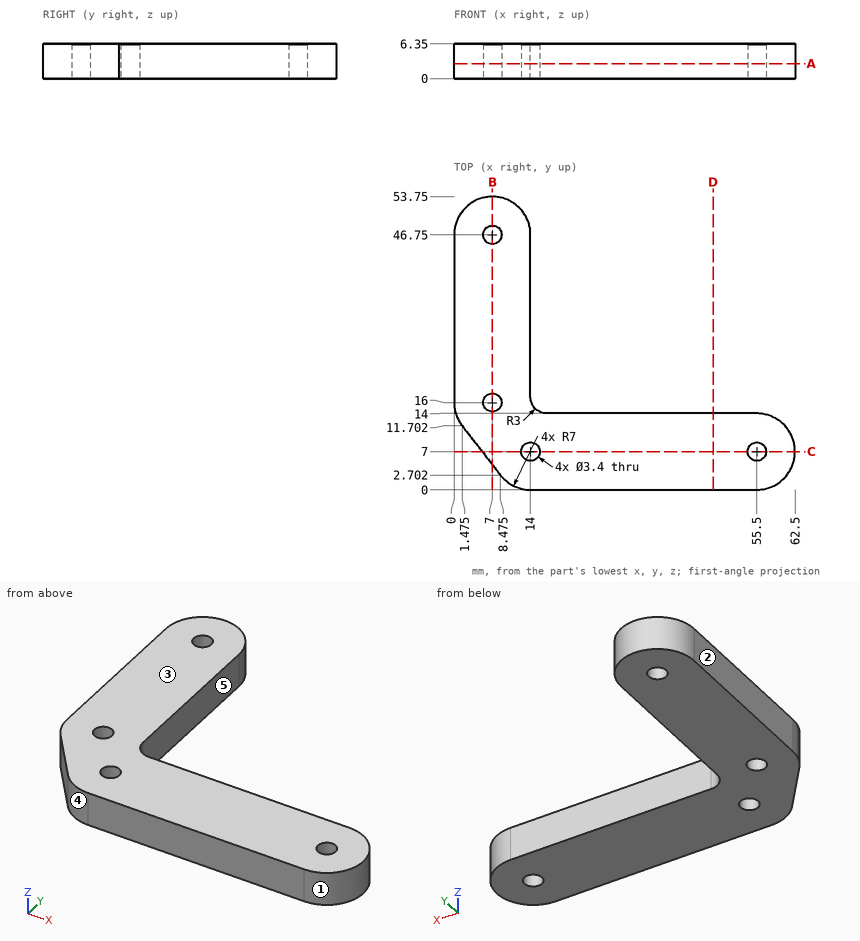
Answer from the drawing. Dimensions are ordinates in mm from the lowest x, y and z of the part. A direction names the side the tool comes from. Coordinates: 2 decimals unless noted, no trailing zeros. Write each loop counter-clockwise with the first axis right and the second up, starting at its lowest first coordinate (ties: lowest second). Pieces come first, ordered by that corner, then holes. Notation, with made-up numbers: M 38,49 L 61,49 A12 ccw 61,56 Z; hole C 38,88.5 d9. An arc over 180 degrees is marked long. Put each result on its own line as item: value. Start each with the question number.
1. Consider line 1 (Y direction, x = 32.5, z = 1.5); line 2 (Y direction, x = 14.5, z = 5) (1 decimal). Determine where each line is inside the solid, lowest interval first. Write a range as from..to.
2. A cutting plane is placed at B-B on x = 7. Write down the section's boundary in (y, z), then the cut area to 3 significant figures.
3. Which of the six approach directions +Z, -Z, +X, -X, +Y, -Y give full straight-line access (tool end or side, diameter ignored) to the marked faces 4 and 5?
4. A flat-ended cylindrical pin translates along its axis: P1, Ø3, axis at x = 26, z = 1, coming from the +Y side. Find the tip coordinate at first contact, or state that the pin passes through.
5. A cutting plane is placed at A-A on z = 2.75. Count the separate pieces of the cut face and the enclosed holes in it, then the cut area to 3 significant figures.
6. A cutting plane is placed at C-C on y = 7. Write down the section's boundary in (x, z).
7. For a pull along X with two mould halves and no side action, classify the marked faces 1, 2 and 3 as pulls with the +X half, pulls with the -X half, needs draft (parallel to the pull), parting line crosses it, or undercut.
8. A cutting plane is placed at D-D on x = 47.5. Write down the section's boundary in (y, z), then the cut area to 3 significant figures.
Resolved:
1. line 1: y = 0..14
1. line 2: y = 0..5.4, 8.6..15.3
2. outline: M 4.6,0 L 14.3,0 L 14.3,6.35 L 4.6,6.35 Z; M 17.7,0 L 45.05,0 L 45.05,6.35 L 17.7,6.35 Z; M 48.45,0 L 53.75,0 L 53.75,6.35 L 48.45,6.35 Z
2. area: 269 mm2
3. face 4: +Z, -Z, -X, -Y
3. face 5: +Z, -Z, +X, +Y
4. P1: stops at y = 14
5. separate pieces: 1
5. enclosed holes: 4
5. area: 1,280 mm2
6. outline: M 5.13,0 L 12.3,0 L 12.3,6.35 L 5.13,6.35 Z; M 15.7,0 L 53.8,0 L 53.8,6.35 L 15.7,6.35 Z; M 57.2,0 L 62.5,0 L 62.5,6.35 L 57.2,6.35 Z
7. face 1: pulls with the +X half
7. face 2: pulls with the -X half
7. face 3: needs draft
8. outline: M 0,0 L 14,0 L 14,6.35 L 0,6.35 Z
8. area: 88.9 mm2
